Geometry: final body of the model. Coordinates: model frame, mm. A direction names the side the tool comes from. Round coordinates to 2 decimals unless told otherwise and drop trailing zeros. Loops run counter-clockwise (first coordinate to the right, second up) from the corner with the lowest first, then second, coordinate; pieces in that order, holes last. Notation, with made-up numbers: (33.25, -16) - (67.25, -16) arc R12 ccw to (67.25, 1) - close; hole circle Ø3 at (6.5, 70.25). An arc over 180 degrees is marked (long way). Return JSON: item names as keys, results as strings. Group by question number.
1. Section C-C on z = 6. Return loops of the section in (x, y).
2. Section D-D on x = -4. Return loops of the section in (y, z).
3. Set-up query: faces 1 (the face through (3.233, 1.341, -2.712)), 2 (the face through (0, -3, 6.6)), 3 (the face through (-0.59, 4.46, 5.08)). Return all of +Z, -Z, +X, -X, +Y, -Y with unobstructed straight access to the full face (end or side cutting, diameter ignored); none if empty.
4. Material intervals for probe 1 along Y at (x, z) = (0, -2); probe 2 along Y at (x, z) = (0, 4.25); probe 3 along Z at (x, y) = (-7.5, 13), sorted ascending.
5. First-contact query: pin 1 Ø4 at (x, z) = (-7.5, 3.5) entering from -Y; pin 2 Ø4 at (x, z) = (-11.5, -1) entering from -Y; pin 3 Ø8 at (x, y) = (6, 12.5) entering from -Z; pin 4 Ø5 at (x, z) = (12, -3) entering from -Y. Flat tips, straight axial feed; report the tip coordinate or a pass-through.
6. Section A-A on y = 0. Return loops of the section in (x, z), and give its area (3 significant figures).
from build123d import *

# Parameters (mm, degrees)
SKETCH_R     = 16.75
PAD_DEPTH    = 3.6
SKETCH003_R  = 3.5
PAD002_DEPTH = 5.5
SKETCH001_R  = 4.5
PAD001_DEPTH = 3
SKETCH002_R  = 2.75
POCKET_DEPTH = 12.101


with BuildPart() as part:
    # Sketch → Pad (new body)
    with BuildSketch(Plane.XY):
        Circle(SKETCH_R)
    extrude(amount=PAD_DEPTH)

    # Sketch003 (on Face2 of Pocket) → Pad002 (join)
    with BuildSketch(Plane(origin=(0, 0, 0), x_dir=(1, 0, 0), z_dir=(0, 0, -1))):
        Circle(SKETCH003_R)
    extrude(amount=PAD002_DEPTH)

    # Sketch001 (on Face3 of Pad) → Pad001 (join)
    with BuildSketch(Plane.XY.offset(3.6)):
        Circle(SKETCH001_R)
    extrude(amount=PAD001_DEPTH)

    # Sketch002 (on Face5 of Pad001) → Pocket (cut, through all)
    with BuildSketch(Plane.XY.offset(6.6)):
        Circle(SKETCH002_R)
    extrude(amount=-POCKET_DEPTH, mode=Mode.SUBTRACT)


solid = part.part
Taken from the geometry:
{
 "1": {"outline": "circle Ø9 at (0, 0); hole circle Ø5.5 at (0, 0)"},
 "2": {"outline": "(-16.27, 0) - (16.27, 0) - (16.27, 3.6) - (2.06, 3.6) - (2.06, 6.6) - (-2.06, 6.6) - (-2.06, 3.6) - (-16.27, 3.6) - close"},
 "3": {"face 1": "-Z", "face 2": "+Z, +X, -X, +Y, -Y", "face 3": "+Z"},
 "4": {"probe 1": "-3.5 to -2.75, 2.75 to 3.5", "probe 2": "-4.5 to -2.75, 2.75 to 4.5", "probe 3": "0 to 3.6"},
 "5": {"pin 1": "y = -15.82", "pin 2": "y = -13.61", "pin 3": "z = 0", "pin 4": "through"},
 "6": {"outline": "(-16.75, 0) - (-3.5, 0) - (-3.5, -5.5) - (-2.75, -5.5) - (-2.75, 6.6) - (-4.5, 6.6) - (-4.5, 3.6) - (-16.75, 3.6) - close; (2.75, -5.5) - (3.5, -5.5) - (3.5, 0) - (16.75, 0) - (16.75, 3.6) - (4.5, 3.6) - (4.5, 6.6) - (2.75, 6.6) - close", "area": "120 mm2"}
}
